```python
from build123d import *

# Parameters (mm, degrees)
SKETCH_1_R               = 5
EXTRUDE_1_DEPTH          = 15
SKETCH_2_W               = 1
SKETCH_2_H               = 10
CUT_EXTRUDE_1_DEPTH      = 2
CUT_EXTRUDE_2_DEPTH      = 5
CUT_EXTRUDE_2_DEPTH_BACK = 5
SKETCH_3_R               = 3


with BuildPart() as part:
    # Sketch 1 → Extrude 1 (new body)
    with BuildSketch(Plane(origin=(0, 0, 0), x_dir=(1, 0, 0), z_dir=(0, 1, 0))):
        with Locations(Location((0, 0, 0), (0, 0, 270))):
            Circle(SKETCH_1_R)
    extrude(amount=EXTRUDE_1_DEPTH)

    # Sketch 2 → Cut-Extrude 1 (cut)
    with BuildSketch(Plane(origin=(0, 15, 0), x_dir=(1, 0, 0), z_dir=(0, 1, 0))):
        Rectangle(SKETCH_2_W, SKETCH_2_H)
    extrude(amount=-CUT_EXTRUDE_1_DEPTH, mode=Mode.SUBTRACT)

    # Sketch 3 → Cut-Extrude 2 (cut, two sides: drawn at the far end of the back side and taken through both)
    with BuildSketch(Plane.XY.offset(-CUT_EXTRUDE_2_DEPTH_BACK)):
        with Locations(Location((0, 7.5, 0), (0, 0, 99.594070543))):
            Circle(SKETCH_3_R)
    extrude(amount=CUT_EXTRUDE_2_DEPTH + CUT_EXTRUDE_2_DEPTH_BACK, mode=Mode.SUBTRACT)


solid = part.part
```
The model under review builds one solid part; all positions refer to its coordinate system, in mm. A direction names the side the tool comes from. Give positions to 0.01 mm unless a question says otherwise; leave off trailing zeros. Order: outer loops, then holes, each group sorted by start corner. A loop starts at its lowest first (then second) coordinate and runs counter-clockwise, first axis right, second up. Notation, with made-up numbers: (-24.75, 23.25) - (-17.75, 23.25) arc R10 cw to (-17.75, 41.25) - close; hole circle Ø5 at (-5.5, 13). An arc over 180 degrees is marked (long way). Use CSV: the item, a comma, the result in double quotes. Start each with the question number.
Q1. To check wall thickness, follow line 1 along Y through (x, z) = (0, -2); line 2 along X through (y, z) = (7.5, 2); line 3 along Y through (x, z) = (1.5, -4). State the ranges of each line that lie inside material, in increasing order. Write a range as [from, to].
Q2. We need section A-A, the plane x = 0. Write out the cut boundary in (y, z).
Q3. Clearance check with flat-ended pins moving along their axes: pin 1 Ø1 at (y, z) = (8, 1.5) entering from +X; pin 2 Ø1.6 at (y, z) = (14.5, -2) entering from -X. State where each tip first meets the part, or that it passes through.
Q4. We need section C-C, the plane z = 1.75. Write out the cut boundary in (x, y), and give its area (3 significant figures).
Q5. The part is to be moulded in two halves that separate along Y. For faces 1 (the flat face through (2, 15, 0)), 2 (the cylindrical face through (2.996, 7.347, -0.07)), 3 (the flat face through (0, 0, 0)), 4 (the flat face through (0.5, 14, 0)), say which applies: +Y half, -Y half, draft (parallel to the pull), parting line (faces both ways), or undercut.
Q6. We need section D-D, the plane y = 7.5. Write out the cut boundary in (x, z).
Q7. Tool access review of faces 5 (the cylindrical face through (3.379, 7.395, -3.685)), 6 (the flat face through (0, 13, 0)): name each direction out of +Z, -Z, +X, -X, +Y, -Y from which nothing blocks a thin tool from reaching the whole face with its end or side.
Outcome:
1,line 1,"y = [0, 4.5], [10.5, 13]"
1,line 2,"x = [-4.58, -3], [3, 4.58]"
1,line 3,"y = [0, 4.9], [10.1, 15]"
2,outline,"(0, -5) - (4.5, -5) - (4.5, 5) - (0, 5) - close; (10.5, -5) - (13, -5) - (13, 5) - (10.5, 5) - close"
3,pin 1,"stops at x = 4.9"
3,pin 2,"stops at x = -4.85"
4,outline,"(-4.68, 0) - (4.68, 0) - (4.68, 15) - (0.5, 15) - (0.5, 13) - (-0.5, 13) - (-0.5, 15) - (-4.68, 15) - close; hole circle Ø6 at (0, 7.5)"
4,area,"110 mm^2"
5,face 1,"+Y half"
5,face 2,"undercut"
5,face 3,"-Y half"
5,face 4,"draft"
6,outline,"(-3, -4) - (-3, 4) arc R5 ccw to start; (3, -4) arc R5 ccw to (3, 4) - close"
7,face 5,"+Y, -Y"
7,face 6,"+Z, -Z, +Y"
